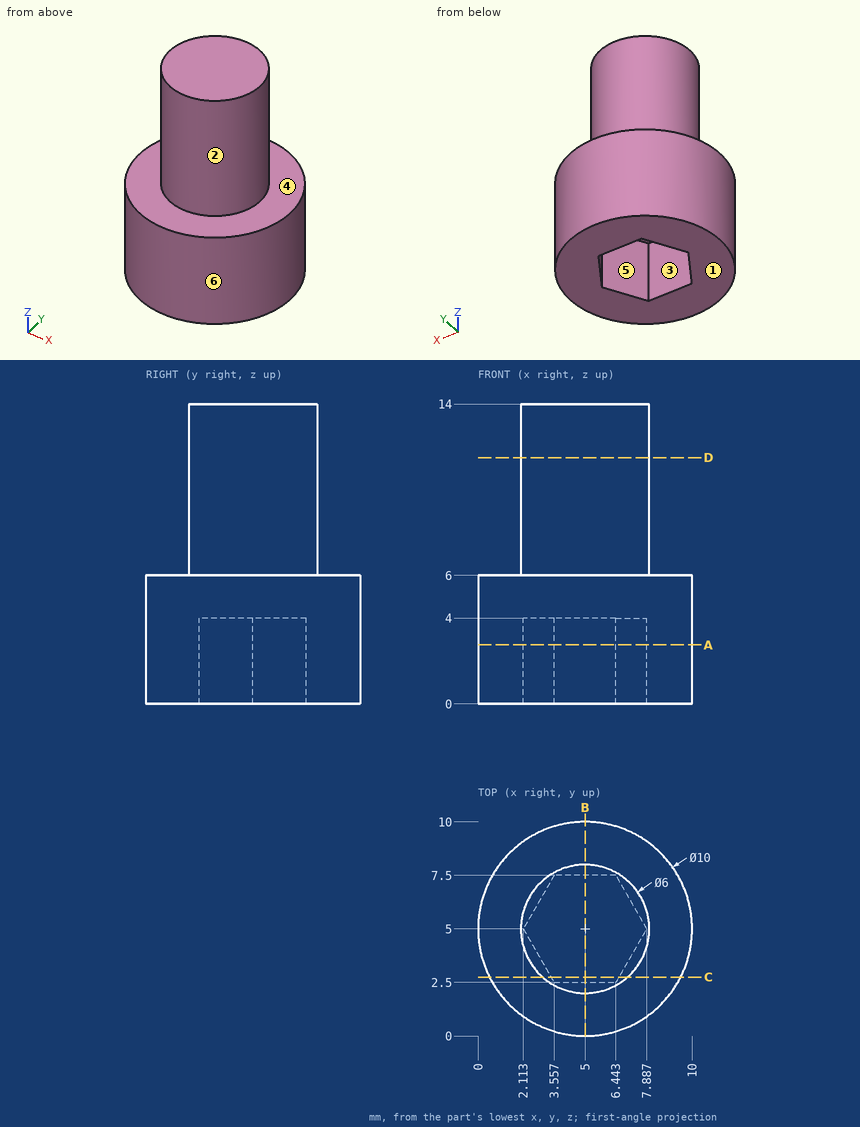
Answer from the drawing. Dimensions are ordinates in mm from the lowest x, y and z of the part. A direction names the side the tool comes from. Coordinates: 2 decimals unless noted, no trailing zeros. Loops run counter-clockwise (first coordinate to the right, second up) from the corner with the lowest first, then second, coordinate; pieces in that order, holes last.
1) Flat-ended cylindrical pins translate along their axes: pin 1 (2 mm diameter, centred on x = 5.5, z = 12, fed in from -Y); pin 2 (1.5 mm diameter, centred on x = 4.5, z = 12, fed in from +Y); pin 3 (1.5 mm diameter, centred on y = 2, z = 8, fed in from -X) (1 decimal). Find the tip coordinate at first contact, or state that the pin passes through.
Results:
pin 1: stops at y = 2
pin 2: stops at y = 8
pin 3: stops at x = 3
2) Section A-A (z = 2.75) is taken. Give the vertices of the cut face in (x, y).
Results:
outline: circle Ø10 at (5, 5); hole (2.11, 5) - (3.56, 2.5) - (6.44, 2.5) - (7.89, 5) - (6.44, 7.5) - (3.56, 7.5) - close
3) Section C-C (y = 2.75) is taken. Give the vertices of the cut face in (x, z) (1 decimal).
Results:
outline: (0.5, 0) - (3.4, 0) - (3.4, 4) - (6.6, 4) - (6.6, 0) - (9.5, 0) - (9.5, 6) - (7, 6) - (7, 14) - (3, 14) - (3, 6) - (0.5, 6) - close
4) Consider probe 1 along Z at (x, y) = (5.5, 1.75); probe 2 along Z at (x, y) = (5, 3.5); probe 3 along X at (y, z) = (9, 0.75). Determine where each line is inside the solid, lowest interval first.
Results:
probe 1: z = 0 to 6
probe 2: z = 4 to 14
probe 3: x = 2 to 8
5) For the marked faces 1, 2 and 3, determine the directions among +Z, -Z, +X, -X, +Y, -Y from which every point of the face is accessible in a straight line to the end or side of a thin tool.
Results:
face 1: -Z, +X, -X, +Y, -Y
face 2: +Z
face 3: -Z
6) Section D-D (z = 11.5) is taken. Give the vertices of the cut face in (x, y).
Results:
outline: circle Ø6 at (5, 5)
7) For a pull along Y with two mould halves and no side action, classify the marked faces 4, 5 and 6 as +Y half, -Y half, draft (parallel to the pull), parting line (faces both ways), or undercut.
Results:
face 4: draft
face 5: undercut
face 6: parting line
8) Section B-B (x = 5) is taken. Give the vertices of the cut face in (y, z), plus the area to 3 significant figures.
Results:
outline: (0, 0) - (2.5, 0) - (2.5, 4) - (7.5, 4) - (7.5, 0) - (10, 0) - (10, 6) - (8, 6) - (8, 14) - (2, 14) - (2, 6) - (0, 6) - close
area: 88.0 mm2
